Part print with two shaded views. Sizes in mm from the minimum x, y, z corner. A direction names the side the tool comes from. Give positions to 0.01 mm unless a question says otherwise; leave off trailing zeros. Write each loop counter-clockwise with the first axis right and the second up, starting at its lowest first coordinate (ties: lowest second). Pieces come first, ordered by that corner, then holes. Notation, with made-up numbers: (-37.5, 14.5) -> (4.5, 14.5) arc R21 cw to (4.5, 20.5) -> close; hole circle Ø7 at (-13.75, 6). An arc over 180 degrees is marked (long way). Answer as a JSON object with one key per item and string values.
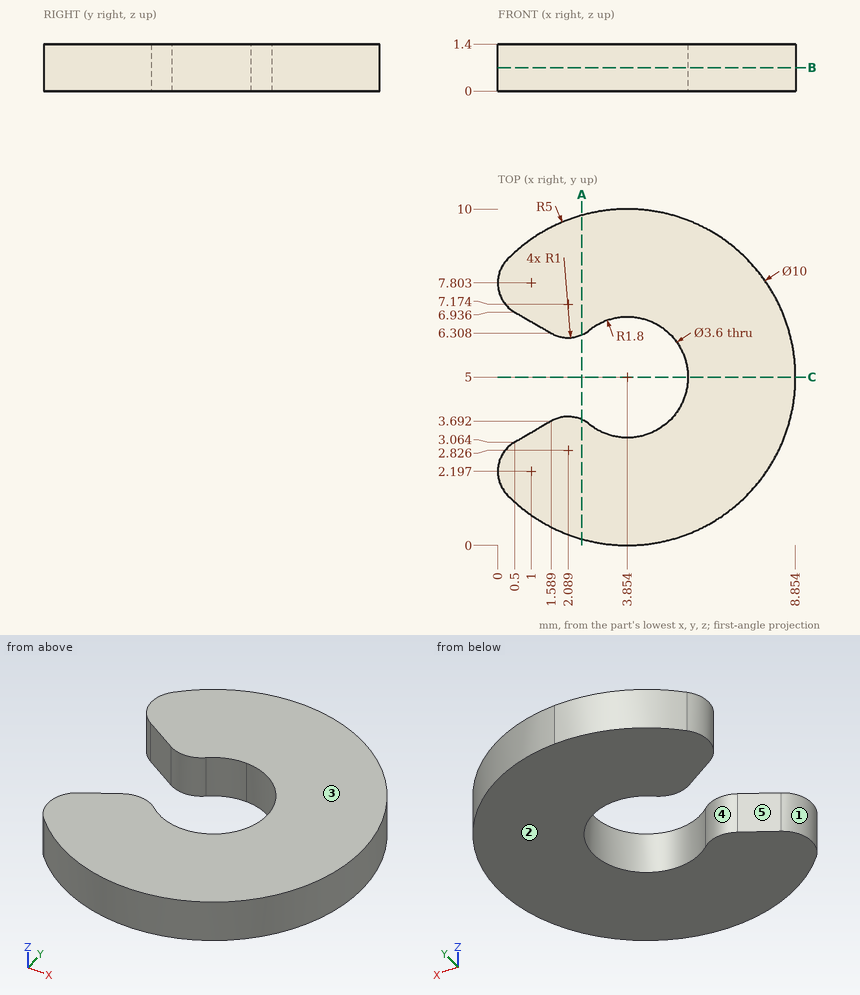
1) Mould opens along Y. For the marked faces 1 and 2 say: released by +Y, released by -Y, zero draft, split by the parting line, or undercut.
Model answer:
{"face 1": "undercut", "face 2": "zero draft"}
2) Slice it at A-A (x = 2.5). List the corners of the cut face in (y, z).
Model answer:
{"outline": "(0.19, 0) -> (3.74, 0) -> (3.74, 1.4) -> (0.19, 1.4) -> close; (6.26, 0) -> (9.81, 0) -> (9.81, 1.4) -> (6.26, 1.4) -> close"}
3) 3-axis set-ups, long thin cutter, end or side, ignore diameter. For the marked faces 3, 4 and 5: which of +Z, -Z, +X, -X, +Y, -Y reach the whole face in a straight line?
Model answer:
{"face 3": "+Z, +X, -X, +Y, -Y", "face 4": "+Z, -Z", "face 5": "+Z, -Z, -X"}
4) Slice it at C-C (y = 5). List the corners of the cut face in (x, z) (1 decimal).
Model answer:
{"outline": "(5.7, 0) -> (8.9, 0) -> (8.9, 1.4) -> (5.7, 1.4) -> close"}
5) Wall check: probe 1 along X at (y, z) = (5, 0.75) (1 decimal); probe 2 along Y at (x, z) = (2.25, 0.3) (1 decimal); probe 3 along Y at (x, z) = (2.5, 0.85) (1 decimal). Give the ranges that are in metal, low to high.
Model answer:
{"probe 1": "x = 5.7 to 8.9", "probe 2": "y = 0.3 to 3.8, 6.2 to 9.7", "probe 3": "y = 0.2 to 3.7, 6.3 to 9.8"}
6) Slice it at B-B (z = 0.7). List the corners of the cut face in (x, y) (1 decimal).
Model answer:
{"outline": "(0.3, 1.5) arc R5 ccw (long way) to (0.3, 8.5) arc R1 ccw to (0.5, 6.9) -> (1.6, 6.3) arc R1 ccw to (2.7, 6.4) arc R1.8 cw (long way) to (2.7, 3.6) arc R1 ccw to (1.6, 3.7) -> (0.5, 3.1) arc R1 ccw to start"}
